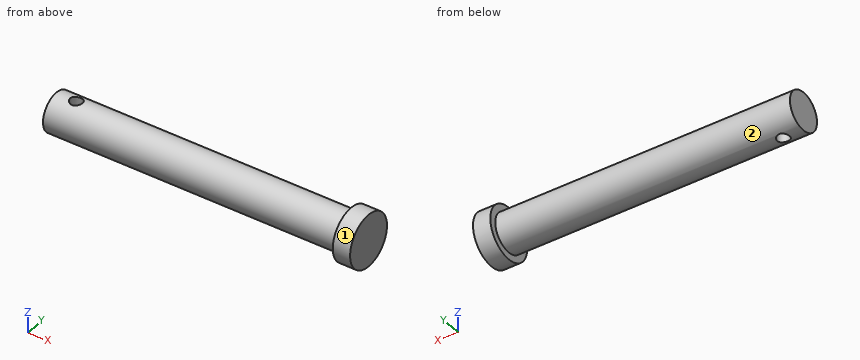
from build123d import *

# Parameters (mm, degrees)
F0_W     = 90
F0_H     = 5.5
F2_R     = 1.75
F3_DEPTH = 15
F4_R     = 7.5
F4_R_2   = 5.5
F5_DEPTH = 5


with BuildPart() as f1:
    # F0 (on Front) → F1 (revolve)
    with BuildSketch(Plane.XZ):
        with Locations((0, 2.75)):
            Rectangle(F0_W, F0_H)
    revolve(axis=Axis((0, 0, 0), (1, 0, 0)))

    # F2 (on Top) → F3 (cut, symmetric)
    with BuildSketch(Plane.XY):
        with Locations((-39.25, 0)):
            Circle(F2_R)
    extrude(amount=F3_DEPTH, both=True, mode=Mode.SUBTRACT)

    # F4 (on face) → F5 (join)
    with BuildSketch(Plane.YZ.offset(45)):
        Circle(F4_R)
        Circle(F4_R_2, mode=Mode.SUBTRACT)
    extrude(amount=-F5_DEPTH)


solid = f1.part
CAD build for the part. Positions are in the model's coordinates, mm. Face numbers are marked on the shaded views. A direction names the side the tool comes from. Coordinates: 2 decimals unless noted, no trailing zeros. Loops run counter-clockwise (first coordinate to the right, second up) from the corner with the lowest first, then second, coordinate; pieces in that order, holes last. Notation, with made-up numbers: (35.5, 41.5) - (63.5, 41.5) arc R20 cw to (63.5, 45.5) - close; hole circle Ø3 at (83.5, -36). An arc over 180 degrees is marked (long way). Use one line per item in the form item = value. Start each with the question number.
1) Band-saw the part on A-A (y = 0). Give the cut face in (x, z), and give its area (4 significant figures).
2) Band-saw the part on B-B (z = 2.5). Give the cut face in (x, y).
3) Flat gauge pins, fed straight in: pin 1 (1 mm diameter, centred on x = -29, z = 3.5, fed in from -Y); pin 2 (3 mm diameter, centred on x = -0.5, z = 3, fed in from -Y); pin 3 (8 mm diameter, centred on x = 29, z = 1, fed in from +Y). Where does each tip first touch, or does it go through?
4) Band-saw the part on D-D (y = 4.5). Give the cut face in (x, z), and give its area (3 significant figures).
5) Tool access for the marked faces 1 and 2: list every direction of +Z, -Z, +X, -X, +Y, -Y with a clear straight run to the whole face (end or side of a thin tool).
6) Drill centre lines: L1, parallel to Y at x = -39.25, z = 2.5; L2, parallel to X at y = 2.5, z = 5.5; L3, parallel to Y at x = -39.25, z = 1. Where is each one in solid material? Low to high. Write a range as from..to.
7) Band-saw the part on C-C (x = -39.25). Give the cut face in (y, z).
Check values:
q1.outline = (-45, -5.5) - (-41, -5.5) - (-41, 5.5) - (-45, 5.5) - close; (-37.5, -5.5) - (40, -5.5) - (40, -7.5) - (45, -7.5) - (45, 7.5) - (40, 7.5) - (40, 5.5) - (-37.5, 5.5) - close
q1.area = 971.5 mm2
q2.outline = (-45, -4.9) - (40, -4.9) - (40, -7.07) - (45, -7.07) - (45, 7.07) - (40, 7.07) - (40, 4.9) - (-45, 4.9) - close; hole circle Ø3.5 at (-39.25, 0)
q3.pin_1 = -4.61
q3.pin_2 = -5.29
q3.pin_3 = 5.5
q4.outline = (-45, -3.16) - (40, -3.16) - (40, -6) - (45, -6) - (45, 6) - (40, 6) - (40, 3.16) - (-45, 3.16) - close
q4.area = 598 mm2
q5.face_1 = +X, -X
q5.face_2 = -X
q6.L1 = -4.9..-1.75, 1.75..4.9
q6.L2 = 40..45
q6.L3 = -5.41..-1.75, 1.75..5.41
q7.outline = (-1.75, -5.21) - (-1.75, 5.21) arc R5.5 ccw to start; (1.75, -5.21) arc R5.5 ccw to (1.75, 5.21) - close
